Geometry: final body of the model. Coordinates: model frame, mm. Coordinates: 2 decimals unless noted, no trailing zeros. Loops run counter-clockwise (first coordinate to the right, second up) from the corner with the lowest first, then second, coordinate; pieces in that order, holes last. Notation, with made-up numbers: (19.25, -18.5) -> (53.25, -18.5) arc R19 cw to (53.25, -2.5) -> close; hole circle Ø5 at (56.25, 23). An arc over 180 degrees is marked (long way). One line per item, written item: value. Start each with the question number.
Item 1: Section query A-A on z = 18. Return loops of the section in (x, y).
Item 2: Contact query for flat-ended pins moving along their axis: pin 1 Ø10 at (x, z) = (40, 13) entering from +Y; pin 2 Ø1 at (y, z) = (-16.5, 30.5) entering from -X; pin 3 Ø12 at (x, y) = (8.5, 4) entering from -Z. Output: stop coordinate, or through.
Item 3: Ray query, probe 1 along X at (y, z) = (-63, 100); probe 2 along Y at (x, z) = (-19.5, -5); probe 3 along Z at (x, y) = (0.5, -27.5). Return the intervals inside material, ascending. Write a range as from..to.
Item 4: Section query C-C on y = -64. Return loops of the section in (x, z).
Item 5: Section query B-B on x = -55. Return loops of the section in (y, z), then the cut area to 3 significant figures.
from build123d import *

# Parameters (mm, degrees)
F0_R     = 75
F1_DEPTH = 2
F2_R     = 75
F3_DEPTH = 2


with BuildPart() as f1:
    # F0 (on Front) → F1 (new body)
    with BuildSketch(Plane.XZ):
        Circle(F0_R)
    extrude(amount=F1_DEPTH)

    # F2 (on Right) → F3 (join)
    with BuildSketch(Plane.YZ):
        with Locations((-2, 74.973329)):
            Circle(F2_R)
    extrude(amount=F3_DEPTH)


solid = f1.part
Reply:
1. outline: (-72.81, -2) -> (0, -2) -> (0, -50.78) -> (2, -50.78) -> (2, -2) -> (72.81, -2) -> (72.81, 0) -> (2, 0) -> (2, 46.78) -> (0, 46.78) -> (0, 0) -> (-72.81, 0) -> close
2. pin 1: stops at y = 0
2. pin 2: stops at x = 0
2. pin 3: stops at z = -74.89
3. probe 1: x = 0..2
3. probe 2: y = -2..0
3. probe 3: z = 4.44..145.51
4. outline: (0, 32.77) -> (2, 32.77) -> (2, 117.18) -> (0, 117.18) -> close
5. outline: (-2, -50.99) -> (0, -50.99) -> (0, 50.99) -> (-2, 50.99) -> close
5. area: 204 mm²
